Work out the finished part from the listing and answer in its coordinate system (mm). Give positions to 0.01 mm unless a question says otherwise; leave off trailing zeros. Loops run counter-clockwise (first coordinate to the right, second up) from the corner with the lowest first, then second, coordinate; pieces in that order, holes last. Notation, with made-up numbers: (4.25, 21) -> (25.25, 21) arc R12 cw to (25.25, 30) -> close; hole circle Ø8 at (-9, -16.5). An arc over 180 degrees is marked (long way). Answer as CSV lines item,"result". Start each with the question number.
1. Find section C-C, the plane z = 27.5. Give the vertices of the cut face in (x, y).
2. Find the intervals of material crossed by line 1 along Y through (x, z) = (0, 63); line 2 along Y through (x, z) = (-0.5, 20.5); line 3 along X through (y, z) = (14, 64), in increasing order.
3. Find section D-D, the plane z = 61.5. Give the vertices of the cut face in (x, y), and give its area (3 significant figures).
4. Find section B-B, the plane y = -2.5. Give the vertices of the cut face in (x, z), and give its area (3 significant figures).
5. Find section A-A, the plane x = 0. Give the vertices of the cut face in (y, z), and give its area (3 significant figures).
6. Flat-ended cylindrical pins translate along their axes: pin 1 Ø10 at (x, y) = (12.5, -8.5) entering from -Z; pin 2 Ø2 at (y, z) = (-17, 21.5) entering from +X; pin 3 Ø3 at (x, y) = (-1.5, 1.5) entering from +Z; pin 4 Ø6 at (x, z) = (14, 33) entering from +Y. Find the tip coordinate at first contact, or state that the pin passes through.
from build123d import *

# Parameters (mm, degrees)
SKETCH_1_R          = 22.5
EXTRUDE_1_DEPTH     = 70
SKETCH_2_R          = 2
CUT_EXTRUDE_1_DEPTH = 10
SKETCH_5_R          = 5
CUT_EXTRUDE_2_DEPTH = 5


with BuildPart() as part:
    # 草图1 → 凸台-拉伸1 (new body)
    with BuildSketch(Plane.XY):
        Circle(SKETCH_1_R)
    extrude(amount=EXTRUDE_1_DEPTH)

    # 草图2 → 切除-拉伸1 (cut)
    with BuildSketch(Plane.XY.offset(70)):
        with Locations((0, 14.5)):
            Circle(SKETCH_2_R)
        with Locations((0, -14.5)):
            Circle(SKETCH_2_R)
    extrude(amount=-CUT_EXTRUDE_1_DEPTH, mode=Mode.SUBTRACT)

    # 草图5 → 切除-拉伸2 (cut)
    with BuildSketch(Plane.XY.offset(70)):
        Circle(SKETCH_5_R)
    extrude(amount=-CUT_EXTRUDE_2_DEPTH, mode=Mode.SUBTRACT)


solid = part.part
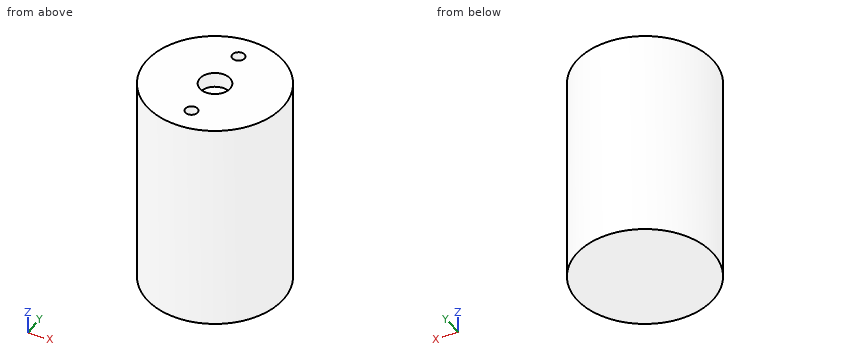
Resolved:
1,outline,"circle Ø45 at (0, 0)"
2,line 1,"y = -22.5 to -16.5, -12.5 to 12.5, 16.5 to 22.5"
2,line 2,"y = -22.49 to 22.49"
2,line 3,"x = -17.61 to -1.94, 1.94 to 17.61"
3,outline,"circle Ø45 at (0, 0); hole circle Ø4 at (0, -14.5); hole circle Ø4 at (0, 14.5)"
3,area,"1,570 mm^2"
4,outline,"(-22.36, 0) -> (22.36, 0) -> (22.36, 70) -> (4.33, 70) -> (4.33, 65) -> (-4.33, 65) -> (-4.33, 70) -> (-22.36, 70) -> close"
4,area,"3,090 mm^2"
5,outline,"(-22.5, 0) -> (22.5, 0) -> (22.5, 70) -> (16.5, 70) -> (16.5, 60) -> (12.5, 60) -> (12.5, 70) -> (5, 70) -> (5, 65) -> (-5, 65) -> (-5, 70) -> (-12.5, 70) -> (-12.5, 60) -> (-16.5, 60) -> (-16.5, 70) -> (-22.5, 70) -> close"
5,area,"3,020 mm^2"
6,pin 1,"stops at z = 0"
6,pin 2,"stops at x = 15.82"
6,pin 3,"stops at z = 65"
6,pin 4,"stops at y = 19.63"
